```python
from build123d import *

# Parameters (mm, degrees)
SKETCH5_W          = 3.8
SKETCH5_H          = 0.5
SKETCH5_W_2        = 0.5
SKETCH5_H_2        = 3.8
CUT_EXTRUDE2_DEPTH = 0.25


with BuildPart() as part:
    # Sketch4 → Revolve1 (revolve)
    with BuildSketch(Plane(origin=(0, 0, 0), x_dir=(0, 0, -1), z_dir=(1, 0, 0)), mode=Mode.PRIVATE) as revolve1_sk:
        Polygon((0, 0), (0, 2.8), (1.65, 1.5), (6, 1.5), (6, 0), align=None)
    revolve(revolve1_sk.sketch.rotate(Axis((0, 0, 0), (0, 0, -1)), 90), axis=Axis((0, 0, 0), (0, 0, -1)))

    # Sketch5 → Cut-Extrude2 (cut)
    with BuildSketch(Plane.XY):
        Rectangle(SKETCH5_W, SKETCH5_H)
        Rectangle(SKETCH5_W_2, SKETCH5_H_2)
    extrude(amount=-CUT_EXTRUDE2_DEPTH, mode=Mode.SUBTRACT)


solid = part.part
```
The model under review builds one solid part; all positions refer to its coordinate system, in mm. Coordinates: 2 decimals unless noted, no trailing zeros. Write each loop counter-clockwise with the first axis right and the second up, starting at its lowest first coordinate (ties: lowest second). Pieces come first, ordered by that corner, then holes.
1) We need section C-C on z = -2.75. State the section outline as (x, y) points, then the cut area to 3 significant figures.
2) We need section D-D on z = -1.25. State the section outline as (x, y) points, then the cut area to 3 significant figures.
3) We need section A-A on y = 0. State the section outline as (x, z) points, then the cut area to 3 significant figures.
4) The part is to be moulded in two halves that separate along Y. For faces 1 (the face through (0, 0, -0.25)), 2 (the face through (-1, 1, 0)), 3 (the face through (1.43, -0.45, -3.86)), say which applies: pulls with the +Y half, pulls with the -Y half, needs draft (parallel to the pull), parting line crosses it, or undercut.
5) To check wall thickness, follow probe 1 along X at (y, z) = (0.05, -2.75); probe 2 along Z at (x, y) = (-0.65, 0.1); probe 3 along Z at (x, y) = (2.3, -0.75). State the ranges of each line that lie inside material, in increasing order.
6) Clearance check with a flat-ended pin moving along its axis: pin 1 Ø2 at (y, z) = (-1.5, -3.5) entering from +X. State where the tip first meets the part, or that it passes through.
Answer list:
1. outline: circle Ø3 at (0, 0)
1. area: 7.07 mm2
2. outline: circle Ø3.63 at (0, 0)
2. area: 10.4 mm2
3. outline: (-2.8, 0) - (-1.5, -1.65) - (-1.5, -6) - (1.5, -6) - (1.5, -1.65) - (2.8, 0) - (1.9, 0) - (1.9, -0.25) - (-1.9, -0.25) - (-1.9, 0) - close
3. area: 19.2 mm2
4. face 1: undercut
4. face 2: needs draft
4. face 3: parting line crosses it
5. probe 1: x = -1.5 to 1.5
5. probe 2: z = -6 to -0.25
5. probe 3: z = -0.48 to 0
6. pin 1: stops at x = 1.41
